Here's the drawing with two shaded views (mm, measured from the low corner). I have some questions. Round coordinates to 2 decimals unless told otherwise and drop trailing zeros. Loops run counter-clockwise (first coordinate to the right, second up) from the corner with the lowest first, then second, coordinate; pieces in that order, holes last.
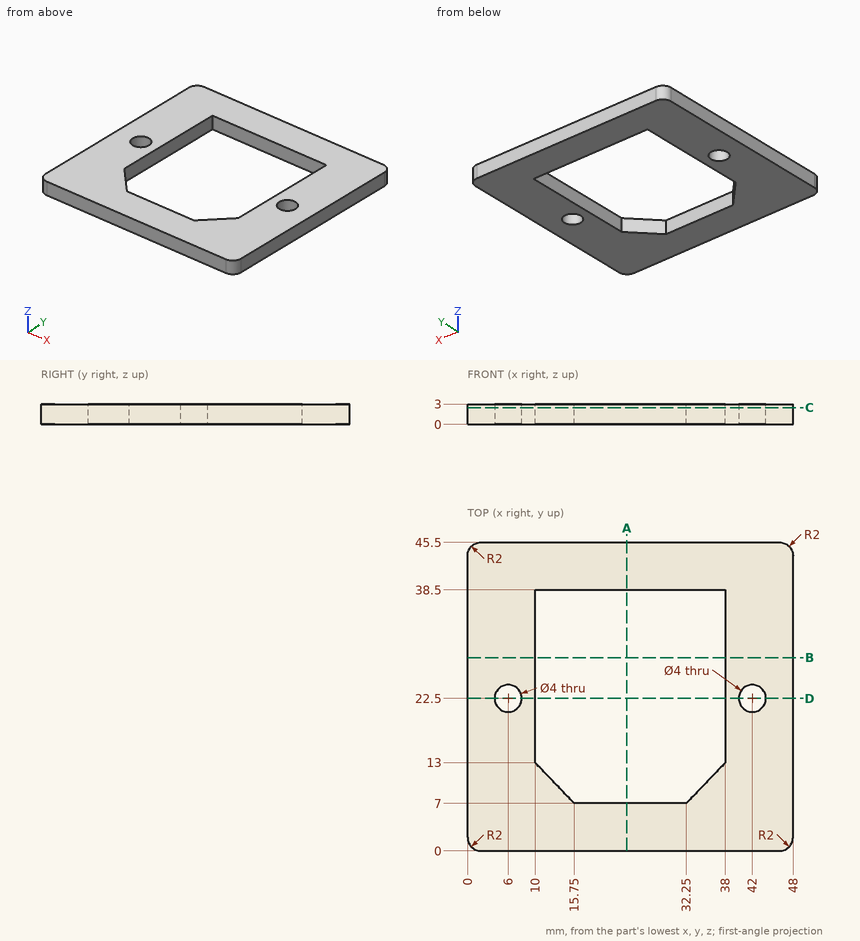
(1) Will this pin go through, and if not, where does the flat tip stop? P1, Ø2.5, axis at x = 42, y = 22.5, coming from the +Z side.
Worked answers:
P1: passes through
(2) If we section it at C-C, the plane z = 2.45: List the corners of the cut face in (x, y) for me, then the cut area to 3 significant figures.
Worked answers:
outline: (0, 2) arc R2 ccw to (2, 0) - (46, 0) arc R2 ccw to (48, 2) - (48, 43.5) arc R2 ccw to (46, 45.5) - (2, 45.5) arc R2 ccw to (0, 43.5) - close; hole circle Ø4 at (6, 22.5); hole (10, 13) - (15.75, 7) - (32.25, 7) - (38, 13) - (38, 38.5) - (10, 38.5) - close; hole circle Ø4 at (42, 22.5)
area: 1,310 mm2
(3) If I drill on line 1 (X direction, y = 33.5, z = 2.1); line 2 (Y direction, x = 6, z = 0.7); line 3 (Y direction, x = 26.5, z = 2.4), over which ranges is the centre line in solid material (lowest first)?
Worked answers:
line 1: x = 0 to 10, 38 to 48
line 2: y = 0 to 20.5, 24.5 to 45.5
line 3: y = 0 to 7, 38.5 to 45.5
(4) If we section it at B-B, the plane y = 28.5: List the corners of the cut face in (x, z) for me, then the cut area to 3 significant figures.
Worked answers:
outline: (0, 0) - (10, 0) - (10, 3) - (0, 3) - close; (38, 0) - (48, 0) - (48, 3) - (38, 3) - close
area: 60.0 mm2
(5) If we section it at A-A, the plane x = 23.5: List the corners of the cut face in (y, z) for me, then the cut area to 3 significant figures.
Worked answers:
outline: (0, 0) - (7, 0) - (7, 3) - (0, 3) - close; (38.5, 0) - (45.5, 0) - (45.5, 3) - (38.5, 3) - close
area: 42.0 mm2
(6) If we section it at D-D, the plane y = 22.5: List the corners of the cut face in (x, z) for me, then the cut area to 3 significant figures.
Worked answers:
outline: (0, 0) - (4, 0) - (4, 3) - (0, 3) - close; (8, 0) - (10, 0) - (10, 3) - (8, 3) - close; (38, 0) - (40, 0) - (40, 3) - (38, 3) - close; (44, 0) - (48, 0) - (48, 3) - (44, 3) - close
area: 36.0 mm2
